The model under review builds one solid part; all positions refer to its coordinate system, in mm. Give positions to 0.01 mm unless a question says otherwise; leave off trailing zeros. Order: outer loops, then holes, each group sorted by start corner. A loop starts at its lowest first (then second) coordinate and runs counter-clockwise, first axis right, second up. Notation, with made-up numbers: (3.25, 73.5) -> (23.25, 73.5) arc R21 cw to (23.25, 80.5) -> close; hole circle Ø5 at (-14, 24.25). An arc over 180 degrees is marked (long way). Use one line per item in the form item = value.
```python
from build123d import *

# Parameters (mm, degrees)
PAD_DEPTH              = 6.25
FILLET_R               = 6.5
MIRROR_ROLL_ANGLE      = -179.860318
MIRROR_PITCH_ANGLE     = 1.669328
MIRROR_PLACEMENT_ANGLE = 0.337481


with BuildPart() as body:
    # Sketch → Pad (new body)
    with BuildSketch(Plane.XY):
        Polygon((0, 290), (50, 290), (150, 0), (120, 0), (120, 13.2), (30, 13.2), (30, 0), (0, 0), align=None)
        Polygon((15, 210), (15, 130), (89.30566, 130), (61.719453, 210), align=None, mode=Mode.SUBTRACT)
        Polygon((15, 110), (15, 33.2), (122.684971, 33.2), (96.202212, 110), align=None, mode=Mode.SUBTRACT)
        with BuildLine():
            ThreePointArc((18, 223.25), (14.75, 220), (18, 216.75))
            Line((18, 216.75), (38, 216.75))
            ThreePointArc((38, 216.75), (41.25, 220), (38, 223.25))
            Line((38, 223.25), (18, 223.25))
        make_face(mode=Mode.SUBTRACT)
        with BuildLine():
            ThreePointArc((60.5, 123.25), (57.25, 120), (60.5, 116.75))
            Line((60.5, 116.75), (80.5, 116.75))
            ThreePointArc((80.5, 116.75), (83.75, 120), (80.5, 123.25))
            Line((80.5, 123.25), (60.5, 123.25))
        make_face(mode=Mode.SUBTRACT)
        with BuildLine():
            ThreePointArc((18, 123.25), (14.75, 120), (18, 116.75))
            Line((18, 116.75), (38, 116.75))
            ThreePointArc((38, 116.75), (41.25, 120), (38, 123.25))
            Line((38, 123.25), (18, 123.25))
        make_face(mode=Mode.SUBTRACT)
        with BuildLine():
            ThreePointArc((18, 26.45), (14.75, 23.2), (18, 19.95))
            Line((18, 19.95), (38, 19.95))
            ThreePointArc((38, 19.95), (41.25, 23.2), (38, 26.45))
            Line((38, 26.45), (18, 26.45))
        make_face(mode=Mode.SUBTRACT)
        with BuildLine():
            ThreePointArc((101, 26.45), (97.75, 23.2), (101, 19.95))
            Line((101, 19.95), (121, 19.95))
            ThreePointArc((121, 19.95), (124.25, 23.2), (121, 26.45))
            Line((121, 26.45), (101, 26.45))
        make_face(mode=Mode.SUBTRACT)
        Polygon((18, 280), (18, 230), (54.822902, 230), (37.581522, 280), align=None, mode=Mode.SUBTRACT)
    extrude(amount=PAD_DEPTH)

    # Fillet
    fillet_edges = [body.edges().sort_by_distance(p)[0] for p in [
        (0, 0, 3.125),
        (50, 290, 3.125),
        (0, 290, 3.125),
        (150, 0, 3.125),
        (120, 0, 3.125),
        (30, 0, 3.125),
        (61.719453, 210, 3.125),
        (15, 210, 3.125),
        (96.202212, 110, 3.125),
        (15, 110, 3.125),
        (15, 130, 3.125),
        (15, 33.2, 3.125),
        (122.684971, 33.2, 3.125),
        (89.30566, 130, 3.125),
        (30, 13.2, 3.125),
        (120, 13.2, 3.125),
        (18, 280, 3.125),
        (18, 230, 3.125),
        (37.581522, 280, 3.125),
        (54.822902, 230, 3.125),
    ]]
    fillet(fillet_edges, radius=FILLET_R)


with BuildPart() as body_1:
    # Body placement: moved
    add(body.part.moved(Location((-2, 0, 0))))


with BuildPart() as model_body_mirrored:
    # mirror: instance of Body
    add(body_1.part.mirror(Plane(origin=(159.181488, 124.226166, 5.790833), x_dir=(-0.001618, 0.999999, 0), z_dir=(-0.999887, -0.001617, 0.014919))))


with BuildPart() as model_body_mirrored_1:
    # mirror roll: moved
    add(model_body_mirrored.part.rotate(Axis((0, 0, 0), (1, 0, 0)), MIRROR_ROLL_ANGLE))


with BuildPart() as model_body_mirrored_2:
    # mirror pitch: moved
    add(model_body_mirrored_1.part.rotate(Axis((0, 0, 0), (0, 1, 0)), MIRROR_PITCH_ANGLE))


with BuildPart() as model_body_mirrored_3:
    # mirror placement: moved
    add(model_body_mirrored_2.part.moved(Location((-113.201923, 287.892908, 10.586))).rotate(Axis((-113.201923, 287.892908, 10.586), (0, 0, 1)), MIRROR_PLACEMENT_ANGLE))


solid = model_body_mirrored_3.part
```
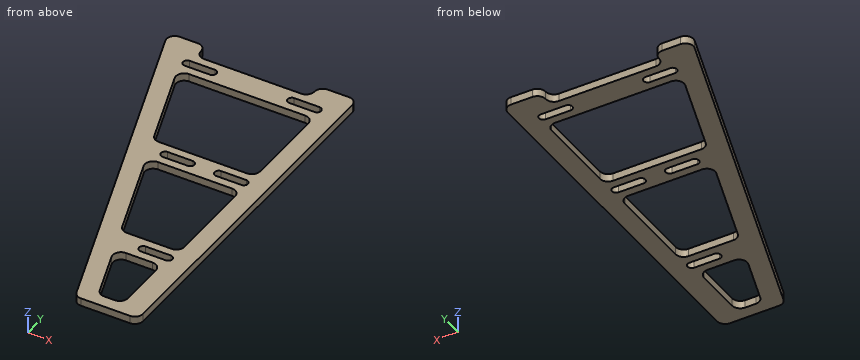
1. Add section C-C on y = 36.5. Give the boundary of the cut face in (x, z), then the cut area to 3 significant figures.
Values:
outline = (145.07, 5.41) -> (145.08, -0.84) -> (160.96, -0.83) -> (160.95, 5.42) -> close; (189.97, 5.44) -> (189.98, -0.81) -> (207.98, -0.8) -> (207.97, 5.45) -> close
area = 212 mm^2
2. Add section B-B on z = 3.25. Count the separate pieces of the cut face and the enclosed holes in it, then the cut area to 3 significant figures.
Values:
separate_pieces = 1
enclosed_holes = 8
area = 13,600 mm^2
3. For pin 1 Ø1 at (x, z) = (129, 2) entering from +Y; pin 2 Ø12 at (x, y) = (95, 228.5) entering from -Z; pin 3 Ø3 at (x, y) = (131.5, 79.5) entering from +Z, all flat-tipped, find the tip position at first contact; note any pin that passes through.
Values:
pin_1 = 275.86
pin_2 = -0.43
pin_3 = 5.51
4. Add section A-A on y = 194.5. Give the boundary of the cut face in (x, z), then the cut area to 3 significant figures.
Values:
outline = (90.13, 5.75) -> (90.14, -0.5) -> (106.02, -0.49) -> (106.01, 5.76) -> close; (192.56, 5.82) -> (192.57, -0.43) -> (207.57, -0.42) -> (207.56, 5.83) -> close
area = 193 mm^2
5. For L1, parallel to X at y = 90, z = 1.5; L2, parallel to X at y = 96.5, z = 3.75; L3, parallel to Z at x = 184, y = 59.5, list the stretches that pass through material, from the lowest coordinate up.
Values:
L1 = 126.47 to 142.36, 192.84 to 207.84
L2 = 124.21 to 140.09, 192.82 to 207.82
L3 = -0.76 to 5.49
